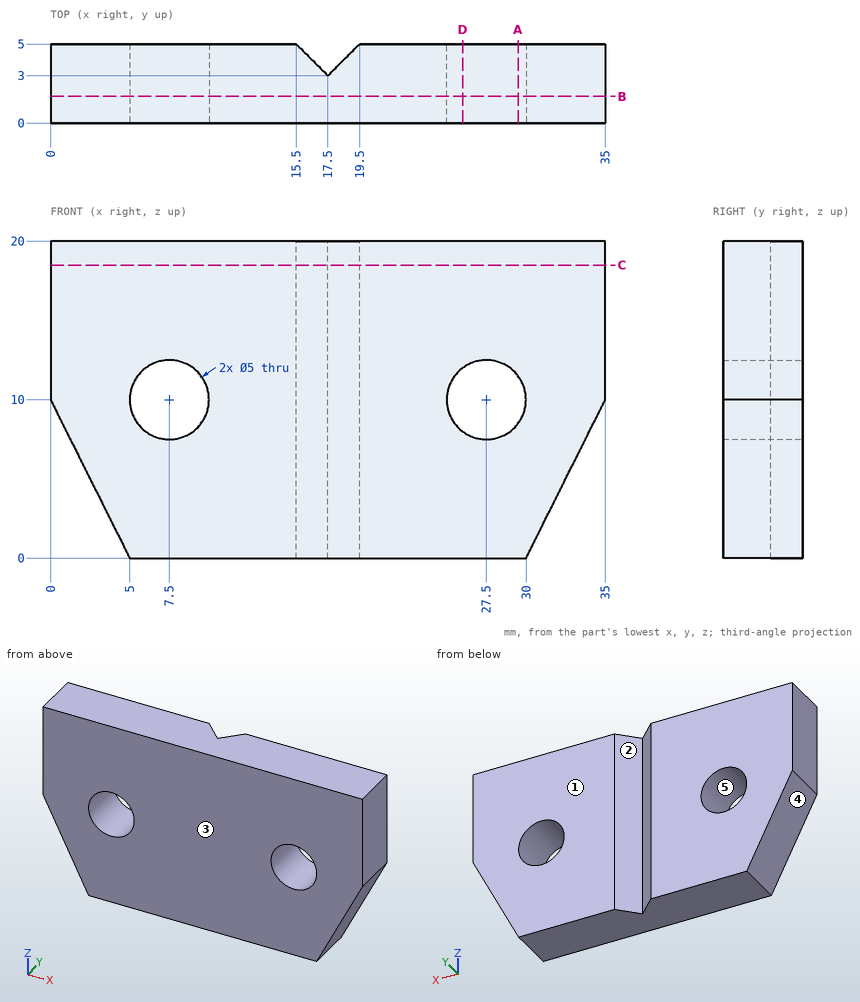
Design review of the part shown in the three views and the two pictorial views. Dimensions are in mm from the part's minimum x, y and z. A direction names the side the tool comes from. Coordinates: 2 decimals unless noted, no trailing zeros. Order: outer loops, then holes, each group sorted by start corner. A loop starts at its lowest first (then second) coordinate and runs counter-clockwise, first axis right, second up. Notation, with made-up numbers: (30.25, 52.25) - (42.25, 52.25) arc R11 cw to (42.25, 59.25) - close; hole circle Ø3 at (48.25, 70). An arc over 180 degrees is marked (long way). Answer as CSV lines item,"result". Start each with the question number.
1) Machinability: for the marked faces 1 and 2, which of the approach directions +Z, -Z, +X, -X, +Y, -Y give a long, thin tool a straight path to every point of the face, cutting with its end or side? Answer none if there is none.
2) Add section B-B (y = 1.7). State the section outline as (x, z) points, then the cut area to 3 significant figures.
3) Draft analysis for pull direction X (two halves, no side actions). For the marked faces 3, 4 and 5, state which applies: +X half, -X half, draft (parallel to the pull), parting line (faces both ways), or undercut.
4) Add section A-A (x = 29.5). State the section outline as (y, z) points.
5) Add section D-D (x = 26). State the section outline as (y, z) points.
6) To check wall thickness, follow line 1 along Z through (x, y) = (27.5, 3.55); line 2 along X through (y, z) = (1.7, 8); line 3 along X through (y, z) = (4.35, 18.75). State the ranges of each line that lie inside material, in increasing order. Write a range as [from, to].
7) Add section C-C (z = 18.5). State the section outline as (x, y) points, then the cut area to 3 significant figures.
Result:
1,face 1,"+Z, -Z, +X, -X, +Y"
1,face 2,"+Z, -Z, +Y"
2,outline,"(0, 10) - (5, 0) - (30, 0) - (35, 10) - (35, 20) - (0, 20) - close; hole circle Ø5 at (7.5, 10); hole circle Ø5 at (27.5, 10)"
2,area,"611 mm^2"
3,face 3,"draft"
3,face 4,"-X half"
3,face 5,"undercut"
4,outline,"(0, 0) - (5, 0) - (5, 8.5) - (0, 8.5) - close; (0, 11.5) - (5, 11.5) - (5, 20) - (0, 20) - close"
5,outline,"(0, 0) - (5, 0) - (5, 8) - (0, 8) - close; (0, 12) - (5, 12) - (5, 20) - (0, 20) - close"
6,line 1,"[0, 7.5], [12.5, 20]"
6,line 2,"[1, 6], [9, 26], [29, 34]"
6,line 3,"[0, 16.15], [18.85, 35]"
7,outline,"(0, 0) - (35, 0) - (35, 5) - (19.5, 5) - (17.5, 3) - (15.5, 5) - (0, 5) - close"
7,area,"171 mm^2"
